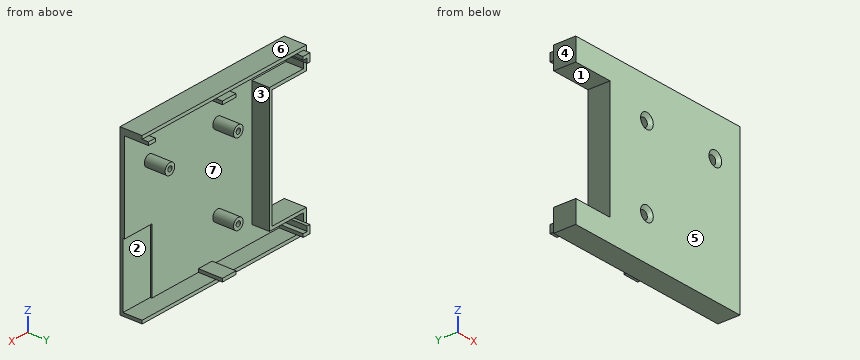
from build123d import *

# Parameters (mm, degrees)
SKETCH_1_W           = 120
SKETCH_1_H           = 101.6
EXTRUDE_1_DEPTH      = 13.8
CUT_EXTRUDE_1_REACH  = 159.839
SKETCH_2_W           = 25
SKETCH_2_H           = 73.6
SKETCH_4_W           = 93
SKETCH_4_H           = 97.6
CUT_EXTRUDE_2_DEPTH  = 11
SKETCH_6_W           = 25
SKETCH_6_H           = 10
CUT_EXTRUDE_3_DEPTH  = 11
SKETCH_7_W           = 5
SKETCH_7_H           = 2
SKETCH_7_W_2         = 10
EXTRUDE_2_DEPTH      = 15
SKETCH_14_W          = 20
SKETCH_14_H          = 40
CUT_EXTRUDE_9_DEPTH  = 16
SKETCH_15_R          = 3.5
EXTRUDE_3_DEPTH      = 13
CUT_EXTRUDE_10_REACH = 160.026
SKETCH_16_R          = 1.6
SKETCH_17_R          = 2.65
CUT_EXTRUDE_11_DEPTH = 8
CHAMFER_1_SIZE       = 2


with BuildPart() as part:
    # 草图1 → 凸台-拉伸1 (new body)
    with BuildSketch(Plane(origin=(0, 0, 0), x_dir=(1, 0, 0), z_dir=(0, 1, 0))):
        with Locations((60, -50.8)):
            Rectangle(SKETCH_1_W, SKETCH_1_H)
    extrude(amount=EXTRUDE_1_DEPTH)

    # 草图2 → 切除-拉伸1 (cut, up to next)
    with BuildSketch(Plane(origin=(0, 13.8, 0), x_dir=(1, 0, 0), z_dir=(0, 1, 0)), mode=Mode.PRIVATE) as cut_extrude_1_sk1:
        with Locations((12.5, -50.8)):
            Rectangle(SKETCH_2_W, SKETCH_2_H)
    cut_extrude_1_tool1 = extrude(cut_extrude_1_sk1.sketch, amount=-CUT_EXTRUDE_1_REACH, mode=Mode.PRIVATE) & part.part
    add(cut_extrude_1_tool1.solids().sort_by_distance((12.5, 13.8, 50.8))[0], mode=Mode.SUBTRACT)

    # 草图4 → 切除-拉伸2 (cut)
    with BuildSketch(Plane(origin=(0, 13.8, 0), x_dir=(1, 0, 0), z_dir=(0, 1, 0))):
        with Locations((73.5, -50.8)):
            Rectangle(SKETCH_4_W, SKETCH_4_H)
    extrude(amount=-CUT_EXTRUDE_2_DEPTH, mode=Mode.SUBTRACT)

    # 草图6 → 切除-拉伸3 (cut)
    with BuildSketch(Plane(origin=(0, 13.8, 0), x_dir=(1, 0, 0), z_dir=(0, 1, 0))):
        with Locations((14.5, -94.6)):
            Rectangle(SKETCH_6_W, SKETCH_6_H)
    cut_extrude_3 = extrude(amount=-CUT_EXTRUDE_3_DEPTH, mode=Mode.SUBTRACT)

    # 镜向1: 切除-拉伸3 across plane
    add(cut_extrude_3.mirror(Plane(origin=(0, 0, 50.8), x_dir=(1, 0, 0), z_dir=(0, 0, -1))), mode=Mode.SUBTRACT)

    # 草图7 → 凸台-拉伸2 (add)
    with BuildSketch(Plane(origin=(0, 2.8, 0), x_dir=(1, 0, 0), z_dir=(0, 1, 0))):
        Polygon((2, -94.6), (4, -94.6), (4, -97.6), (7, -97.6), (7, -99.6), (2, -99.6), align=None)
        with Locations((117.5, -98.6)):
            Rectangle(SKETCH_7_W, SKETCH_7_H)
        with Locations((61, -98.6)):
            Rectangle(SKETCH_7_W_2, SKETCH_7_H)
    extrude_2 = extrude(amount=EXTRUDE_2_DEPTH)

    # 镜向2: 凸台-拉伸2 across plane
    add(extrude_2.mirror(Plane(origin=(0, 0, 50.8), x_dir=(1, 0, 0), z_dir=(0, 0, -1))))

    # 草图14 → 切除-拉伸9 (cut)
    with BuildSketch(Plane(origin=(0, 17.8, 0), x_dir=(1, 0, 0), z_dir=(0, 1, 0))):
        with Locations((110, -22)):
            Rectangle(SKETCH_14_W, SKETCH_14_H)
    extrude(amount=-CUT_EXTRUDE_9_DEPTH, mode=Mode.SUBTRACT)

    # 草图15 → 凸台-拉伸3 (add)
    with BuildSketch(Plane(origin=(0, 2.8, 0), x_dir=(1, 0, 0), z_dir=(0, 1, 0))):
        with Locations(Location((52, -27, 0), (0, 0, 90))):
            Circle(SKETCH_15_R)
        with Locations(Location((52, -77, 0), (0, 0, 90))):
            Circle(SKETCH_15_R)
        with Locations(Location((102, -77, 0), (0, 0, 90))):
            Circle(SKETCH_15_R)
    extrude(amount=EXTRUDE_3_DEPTH)

    # 草图16 → 切除-拉伸10 (cut, up to next)
    with BuildSketch(Plane(origin=(0, 15.8, 0), x_dir=(1, 0, 0), z_dir=(0, 1, 0)), mode=Mode.PRIVATE) as cut_extrude_10_sk1:
        with Locations(Location((52, -27, 0), (0, 0, 270))):
            Circle(SKETCH_16_R)
    cut_extrude_10_tool1 = extrude(cut_extrude_10_sk1.sketch, amount=-CUT_EXTRUDE_10_REACH, mode=Mode.PRIVATE) & part.part
    # 草图16 → 切除-拉伸10 (cut, up to next)
    with BuildSketch(Plane(origin=(0, 15.8, 0), x_dir=(1, 0, 0), z_dir=(0, 1, 0)), mode=Mode.PRIVATE) as cut_extrude_10_sk2:
        with Locations(Location((52, -77, 0), (0, 0, 270))):
            Circle(SKETCH_16_R)
    cut_extrude_10_tool2 = extrude(cut_extrude_10_sk2.sketch, amount=-CUT_EXTRUDE_10_REACH, mode=Mode.PRIVATE) & part.part
    # 草图16 → 切除-拉伸10 (cut, up to next)
    with BuildSketch(Plane(origin=(0, 15.8, 0), x_dir=(1, 0, 0), z_dir=(0, 1, 0)), mode=Mode.PRIVATE) as cut_extrude_10_sk3:
        with Locations(Location((102, -77, 0), (0, 0, 270))):
            Circle(SKETCH_16_R)
    cut_extrude_10_tool3 = extrude(cut_extrude_10_sk3.sketch, amount=-CUT_EXTRUDE_10_REACH, mode=Mode.PRIVATE) & part.part
    add(cut_extrude_10_tool1.solids().sort_by_distance((52, 15.8, 27))[0], mode=Mode.SUBTRACT)
    add(cut_extrude_10_tool2.solids().sort_by_distance((52, 15.8, 77))[0], mode=Mode.SUBTRACT)
    add(cut_extrude_10_tool3.solids().sort_by_distance((102, 15.8, 77))[0], mode=Mode.SUBTRACT)

    # 草图17 → 切除-拉伸11 (cut)
    with BuildSketch(Plane.XZ):
        with Locations(Location((52, 77, 0), (0, 0, 270))):
            Circle(SKETCH_17_R)
        with Locations(Location((52, 27, 0), (0, 0, 90))):
            Circle(SKETCH_17_R)
        with Locations(Location((102, 77, 0), (0, 0, 270))):
            Circle(SKETCH_17_R)
    extrude(amount=-CUT_EXTRUDE_11_DEPTH, mode=Mode.SUBTRACT)

    # 倒角1
    chamfer_1_edges = [part.edges().sort_by_distance(p)[0] for p in [
        (102, 0, 79.65),
        (52, 0, 24.35),
        (52, 0, 79.65),
    ]]
    chamfer(chamfer_1_edges, length=CHAMFER_1_SIZE)


solid = part.part
Check sheet for the modelled part. Datum: model origin and axes. Units: mm. Face numbers are marked on the shaded views. A direction names the side the tool comes from. Give positions to 0.01 mm unless a question says otherwise; leave off trailing zeros. Loops run counter-clockwise (first coordinate to the right, second up) from the corner with the lowest first, then second, coordinate; pieces in that order, holes last. Notation, with made-up numbers: M -16,-32 L 36,-32 A9 cw 36,-28 Z; hole C 55,-38.5 d2. An arc over 180 degrees is marked long. Return JSON: item names as keys, results as strings. Group by question number.
1. Cross-section at D-D on x = 62.5. Record the boundary of the cut face in (y, z).
2. Mould release check, pull along Z, two halves, no side actions. Record for the marked faces 5, 6 and 7: released by +Z, released by -Z, zero draft, split by the parting line, or undercut.
3. Cross-section at A-A on z = 27. Record the boundary of the cut face in (x, y).
4. Tool access check on the marked faces 1, 2, 3 and 4. Record the directions out of +Z, -Z, +X, -X, +Y, -Y that give a thin tool (end or side, any length) a straight path to the whole face; none if there is none.
5. Cross-section at B-B on z = 77. State how many separate pieces and enclosed holes the cut face has, plus the area to 3 significant figures.
6. Go/stop test with flat-tipped pins: pin 1 (2 mm diameter, centred on y = 8, z = 3.5, fed in from +X); pin 2 (3.5 mm diameter, centred on x = 102, z = 77, fed in from -Y); pin 3 (2 mm diameter, centred on y = 11.5, z = 83, fed in from -X). Record where each tip stops, or that it passes through.
7. Thickness scan on L1, parallel to Z at x = 102, y = 10.5; L2, parallel to X at y = 10.5, z = 77; L3, parallel to X at y = 6.4, z = 77. Record the ranges inside material, lowest first.
8. Cross-section at C-C on x = 102. Record the boundary of the cut face in (y, z), plus the area to 3 significant figures.
Return value:
{
 "1": {"outline": "M 0,0 L 13.8,0 L 13.8,2 L 17.8,2 L 17.8,4 L 2.8,4 L 2.8,97.6 L 17.8,97.6 L 17.8,99.6 L 13.8,99.6 L 13.8,101.6 L 0,101.6 Z"},
 "2": {"face 5": "zero draft", "face 6": "released by +Z", "face 7": "undercut"},
 "3": {"outline": "M 25,0 L 47.35,0 L 49.35,2 L 49.35,8 L 50.4,8 L 50.4,15.8 L 48.5,15.8 L 48.5,2.8 L 27,2.8 L 27,13.8 L 25,13.8 Z; M 53.6,8 L 54.65,8 L 54.65,2 L 56.65,0 L 120,0 L 120,1.8 L 100,1.8 L 100,2.8 L 55.5,2.8 L 55.5,15.8 L 53.6,15.8 Z"},
 "4": {"face 1": "-X, +Y, -Y", "face 2": "+X, +Y", "face 3": "+Y", "face 4": "+Z, -Z, -X, +Y, -Y"},
 "5": {"separate pieces": "3", "enclosed holes": "0", "area": "327 mm^2"},
 "6": {"pin 1": "x = 66", "pin 2": "y = 8", "pin 3": "x = 25"},
 "7": {"L1": "0 to 2, 73.5 to 75.4, 78.6 to 80.5, 99.6 to 101.6", "L2": "25 to 27, 48.5 to 50.4, 53.6 to 55.5, 98.5 to 100.4, 103.6 to 105.5", "L3": "25 to 27, 48.5 to 49.35, 54.65 to 55.5, 98.5 to 99.35, 104.65 to 105.5"},
 "8": {"outline": "M 0,0 L 13.8,0 L 13.8,2 L 1.8,2 L 1.8,42 L 2.8,42 L 2.8,73.5 L 15.8,73.5 L 15.8,75.4 L 8,75.4 L 8,74.35 L 2,74.35 L 0,72.35 Z; M 0,81.65 L 2,79.65 L 8,79.65 L 8,78.6 L 15.8,78.6 L 15.8,80.5 L 2.8,80.5 L 2.8,99.6 L 13.8,99.6 L 13.8,101.6 L 0,101.6 Z", "area": "308 mm^2"}
}
